Design review of the part built by this model. Coordinates are the model's own, in mm. Give positions to 0.01 mm unless a question says otherwise; leave off trailing zeros. Write each loop counter-clockwise with the first axis right and the second up, starting at its lowest first coordinate (ties: lowest second). Pieces come first, ordered by that corner, then holes.
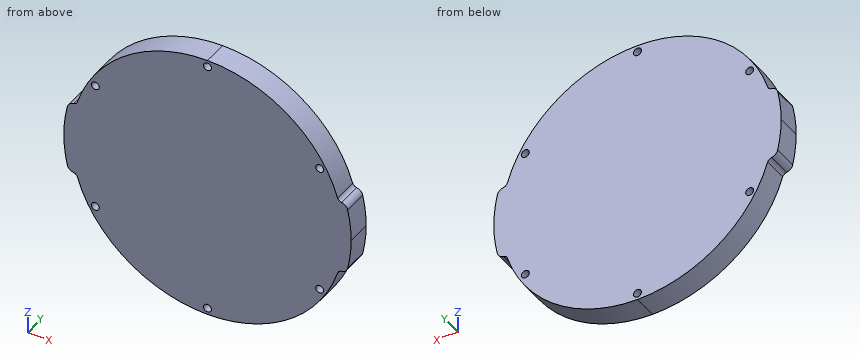
```python
from build123d import *

# Parameters (mm, degrees)
EXTRUDE_1_DEPTH     = 10
FILLET_2_R          = 3
FILLET_3_R          = 2
SKETCH_2_R          = 1.6
CUT_EXTRUDE_1_DEPTH = 11.0000001


with BuildPart() as part:
    # 草图1 → 凸台-拉伸1 (new body)
    with BuildSketch(Plane(origin=(0, 0, 0), x_dir=(1, 0, 0), z_dir=(0, 1, 0))):
        with BuildLine():
            Line((-53.174829572, -15), (-56.285544325, -15))
            ThreePointArc((-56.285544325, -15), (-57.756798115, -7.564044654), (-58.25, 0))
            ThreePointArc((-58.25, 0), (-57.756798115, 7.564044654), (-56.285544325, 15))
            add(Edge.make_bspline(
                [(-56.285544325, 15), (-53.174829572, 15)],
                knots=[0, 0, 1, 1], degree=1))
            ThreePointArc((-53.174829572, 15), (-33.345258284, 44.052880156), (0, 55.25))
            ThreePointArc((0, 55.25), (33.345258284, 44.052880156), (53.174829572, 15))
            Line((53.174829572, 15), (56.285544325, 15))
            ThreePointArc((56.285544325, 15), (57.756798115, 7.564044654), (58.25, 0))
            ThreePointArc((58.25, 0), (57.756798115, -7.564044654), (56.285544325, -15))
            Line((56.285544325, -15), (53.174829572, -15))
            ThreePointArc((53.174829572, -15), (33.345258284, -44.052880156), (0, -55.25))
            ThreePointArc((0, -55.25), (-33.345258284, -44.052880156), (-53.174829572, -15))
        make_face()
    extrude(amount=EXTRUDE_1_DEPTH)

    # 圆角2
    fillet_2_edges = [part.edges().sort_by_distance(p)[0] for p in [
        (-56.285544325, 5, -15),
        (56.285544325, 5, -15),
        (56.285544325, 5, 15),
        (-56.285544325, 5, 15),
    ]]
    fillet(fillet_2_edges, radius=FILLET_2_R)

    # 圆角3
    fillet_3_edges = [part.edges().sort_by_distance(p)[0] for p in [
        (-53.174829572, 5, -15),
        (53.174829572, 5, -15),
        (53.174829572, 5, 15),
        (-53.174829572, 5, 15),
    ]]
    fillet(fillet_3_edges, radius=FILLET_3_R)

    # 草图2 → 切除-拉伸1 (cut, through all)
    with BuildSketch(Plane.XZ):
        with Locations((0, 52.525)):
            Circle(SKETCH_2_R)
        with Locations((45.487984334, 26.2625)):
            Circle(SKETCH_2_R)
        with Locations((45.487984334, -26.2625)):
            Circle(SKETCH_2_R)
        with Locations((0, -52.525)):
            Circle(SKETCH_2_R)
        with Locations((-45.487984334, -26.2625)):
            Circle(SKETCH_2_R)
        with Locations((-45.487984334, 26.2625)):
            Circle(SKETCH_2_R)
    extrude(amount=-CUT_EXTRUDE_1_DEPTH, mode=Mode.SUBTRACT)


solid = part.part
```
(1) To check wall thickness, follow L1, parallel to X at y = 5.75, z = -27.5; L2, parallel to X at y = 5, z = -26; L3, parallel to Z at x = -22.5, y = 4.5. State the ranges of each line that lie inside material, in increasing order.
Resolved:
L1: x = -47.92 to -46.5, -44.47 to 44.47, 46.5 to 47.92
L2: x = -48.75 to -47.07, -43.91 to 43.91, 47.07 to 48.75
L3: z = -50.46 to 50.46
(2) Consider section A-A, the plane y = 8. Give the number of separate pieces and of enclosed holes in the cut face, then the cut area to 3 significant figures.
Resolved:
separate pieces: 1
enclosed holes: 6
area: 9,720 mm2
(3) Consider section C-C, the plane z = -46.5. Give the boundary of the cut face in (x, y).
Resolved:
outline: (-29.84, 0) - (29.84, 0) - (29.84, 10) - (-29.84, 10) - close
(4) Clearance check with flat-ended pins moving along their axes: P1, Ø1.5, axis at x = 13.5, y = 2.5, coming from the +Z side; P2, Ø3, axis at x = 0, z = -52.525, coming from the +Y side (1 decimal); P3, Ø3, axis at y = 5.5, z = -11.5, coming from the -X side; P4, Ø5, axis at y = 5.5, z = -38.5, coming from the -X side. State where each tip first meets the part, or that it passes through.
Resolved:
P1: stops at z = 53.76
P2: passes through
P3: stops at x = -57.39
P4: stops at x = -41.91
(5) Consider section B-B, the plane x = -12. Give the boundary of the cut face in (y, z).
Resolved:
outline: (0, -53.93) - (10, -53.93) - (10, 53.93) - (0, 53.93) - close
